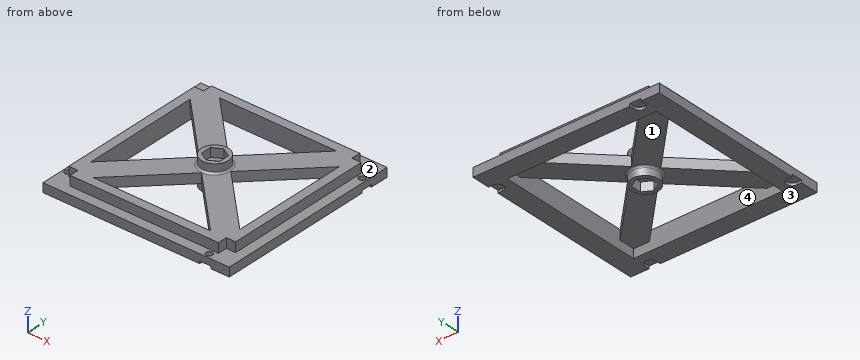
```python
from build123d import *

# Parameters (mm, degrees)
SKETCH_W           = 100
SKETCH_H           = 100
SKETCH_W_2         = 80
SKETCH_H_2         = 80
PAD_DEPTH          = 4.8
SKETCH001_R        = 2.75
PAD001_DEPTH       = 5.2
SKETCH002_R        = 7.25
PAD002_DEPTH       = 4.8
SKETCH003_R        = 7.25
PAD003_DEPTH       = 4.8
POCKET001_DEPTH    = 1.3
SKETCH006_R        = 1.75
POCKET002_DEPTH    = 3.49
POLARPATTERN_COUNT = 4
FILLET_R           = 1


with BuildPart() as part:
    # Sketch → Pad (new body)
    with BuildSketch(Plane.XY):
        Rectangle(SKETCH_W, SKETCH_H)
        Rectangle(SKETCH_W_2, SKETCH_H_2, mode=Mode.SUBTRACT)
    extrude(amount=PAD_DEPTH)

    # Sketch001 (on Face10 of Pad) → Pad001 (join)
    with BuildSketch(Plane.XY.offset(4.8)):
        Polygon((-44.8, 39.8), (-44.8, -39.8), (-39.8, -39.8), (-39.8, -44.8), (39.8, -44.8), (39.8, -39.8), (44.8, -39.8), (44.8, 39.8), (39.8, 39.8), (39.8, 44.8), (-39.8, 44.8), (-39.8, 39.8), align=None)
        Circle(SKETCH001_R, mode=Mode.SUBTRACT)
        Polygon((-31.5, 40), (0, 8.5), (31.5, 40), align=None, mode=Mode.SUBTRACT)
        Polygon((-40, 31.5), (-8.5, 0), (-40, -31.5), align=None, mode=Mode.SUBTRACT)
        Polygon((8.5, 0), (40, 31.5), (40, -31.5), align=None, mode=Mode.SUBTRACT)
        Polygon((0, -8.5), (31.5, -40), (-31.5, -40), align=None, mode=Mode.SUBTRACT)
    extrude(amount=PAD001_DEPTH)

    # Sketch002 (on Face20 of Pad001) → Pad002 (join)
    with BuildSketch(Plane.XY.offset(10)):
        Circle(SKETCH002_R)
        Polygon((0, -5.658033), (4.9, -2.829016), (4.9, 2.829016), (0, 5.658033), (-4.9, 2.829016), (-4.9, -2.829016), align=None, mode=Mode.SUBTRACT)
    extrude(amount=PAD002_DEPTH)

    # Sketch003 (on Face23 of Pad002) → Pad003 (join)
    with BuildSketch(Plane(origin=(0, 0, 4.8), x_dir=(1, 0, 0), z_dir=(0, 0, -1))):
        Circle(SKETCH003_R)
        Polygon((0, -5.658033), (4.9, -2.829016), (4.9, 2.829016), (0, 5.658033), (-4.9, 2.829016), (-4.9, -2.829016), align=None, mode=Mode.SUBTRACT)
    extrude(amount=PAD003_DEPTH)

    # Sketch005 → Pocket001 (cut)
    with BuildSketch(Plane(origin=(0, 0, 0), x_dir=(1, 0, 0), z_dir=(0, 0, -1))):
        with BuildLine():
            ThreePointArc((34.15, 47.5), (37.15, 44.5), (40.15, 47.5))
            Line((40.15, 50), (40.15, 47.5))
            Line((34.15, 50), (40.15, 50))
            Line((34.15, 47.5), (34.15, 50))
        make_face()
    pocket001 = extrude(amount=-POCKET001_DEPTH, mode=Mode.SUBTRACT)

    # Sketch006 (on Face5 of Pocket001) → Pocket002 (cut)
    with BuildSketch(Plane.XY.offset(4.8)):
        with Locations((37.15, -47.5)):
            Circle(SKETCH006_R)
    pocket002 = extrude(amount=-POCKET002_DEPTH, mode=Mode.SUBTRACT)

    # PolarPattern: Pocket002, Pocket001 ×4 about axis
    polarpattern_axis = Axis((0, 0, 4.8), (0, 0, 1))
    for i in range(1, POLARPATTERN_COUNT):
        add(pocket002.rotate(polarpattern_axis, i * 360 / POLARPATTERN_COUNT), mode=Mode.SUBTRACT)
        add(pocket001.rotate(polarpattern_axis, i * 360 / POLARPATTERN_COUNT), mode=Mode.SUBTRACT)

    # Fillet
    fillet_edges = [part.edges().sort_by_distance(p)[0] for p in [
        (-7.25, 0, 10),
        (-7.25, 0, 4.8),
    ]]
    fillet(fillet_edges, radius=FILLET_R)


solid = part.part
```
Input: part model. Units: mm. Frame: model coordinates. Face numbers are marked on the shaded views. A direction names the side the tool comes from. Give positions to 0.01 mm unless a question says otherwise; leave off trailing zeros. Order: outer loops, then holes, each group sorted by start corner. A loop starts at its lowest first (then second) coordinate and runs counter-clockwise, first axis right, second up. Notation, with made-up numbers: (17.5, 42.5) - (75.5, 42.5) arc R28 cw to (75.5, 72.5) - close; hole circle Ø1 at (62, 50.25). An arc over 180 degrees is marked (long way). One line per item, written item: value.
1. Line query: probe 1 along Y at (x, z) = (-37.15, 3.9); probe 2 along Y at (x, z) = (0, 6.2). Output: solid intervals per line, ascending.
Determined:
probe 1: -50 to -40, 40 to 45.75, 49.25 to 50
probe 2: -44.8 to -40, -8.5 to -2.75, 2.75 to 8.5, 40 to 44.8
2. Draft query along X for the marked faces 3 and 4. Return one class per face: released by +X, released by -X, zero draft, split by the parting line, or undercut.
Determined:
face 3: zero draft
face 4: undercut
3. Cut plane B-B, the plane z = 7.75. Output: boundary loops of the cut face in (x, y).
Determined:
outline: (-44.8, -39.8) - (-39.8, -39.8) - (-39.8, -44.8) - (39.8, -44.8) - (39.8, -39.8) - (44.8, -39.8) - (44.8, 39.8) - (39.8, 39.8) - (39.8, 44.8) - (-39.8, 44.8) - (-39.8, 39.8) - (-44.8, 39.8) - close; hole (-40, -31.5) - (-8.5, 0) - (-40, 31.5) - close; hole (-31.5, -40) - (31.5, -40) - (0, -8.5) - close; hole (-31.5, 40) - (0, 8.5) - (31.5, 40) - close; hole circle Ø5.5 at (0, 0); hole (8.5, 0) - (40, -31.5) - (40, 31.5) - close
4. Cut plane D-D, the plane x = 17. Output: boundary loops of the cut face in (y, z).
Determined:
outline: (-50, 0) - (-40, 0) - (-40, 10) - (-44.8, 10) - (-44.8, 4.8) - (-50, 4.8) - close; (-25.5, 4.8) - (-8.5, 4.8) - (-8.5, 10) - (-25.5, 10) - close; (8.5, 4.8) - (25.5, 4.8) - (25.5, 10) - (8.5, 10) - close; (40, 0) - (50, 0) - (50, 4.8) - (44.8, 4.8) - (44.8, 10) - (40, 10) - close
5. Cut plane A-A, the plane x = 37.15. Output: boundary loops of the cut face in (y, z), and give its area (3 significant figures).
Determined:
outline: (-50, 1.3) - (-44.5, 1.3) - (-44.5, 0) - (-40, 0) - (-40, 4.8) - (-28.65, 4.8) - (-28.65, 10) - (-44.8, 10) - (-44.8, 4.8) - (-45.75, 4.8) - (-45.75, 1.31) - (-49.25, 1.31) - (-49.25, 4.8) - (-50, 4.8) - close; (28.65, 4.8) - (40, 4.8) - (40, 0) - (50, 0) - (50, 4.8) - (44.8, 4.8) - (44.8, 10) - (28.65, 10) - close
area: 245 mm2
6. Cut plane C-C, the plane y = 37.15. Output: boundary loops of the cut face in (x, z), and give its area (3 significant figures).
Determined:
outline: (-50, 0) - (-40, 0) - (-40, 4.8) - (-28.65, 4.8) - (-28.65, 10) - (-44.8, 10) - (-44.8, 4.8) - (-50, 4.8) - close; (28.65, 4.8) - (40, 4.8) - (40, 0) - (44.5, 0) - (44.5, 1.3) - (50, 1.3) - (50, 4.8) - (49.25, 4.8) - (49.25, 1.31) - (45.75, 1.31) - (45.75, 4.8) - (44.8, 4.8) - (44.8, 10) - (28.65, 10) - close
area: 245 mm2
7. Reachability of the marked faces 1 and 2 from +Z, -Z, +X, -X, +Y, -Y: full face, straight path, thin tool, end or side. Return the list, or none.
Determined:
face 1: -Z
face 2: +Z
8. Pin query (flat end, axial travel): pin 1 Ø3 at (x, y) = (-47, -37) entering from +Z; pin 2 Ø5.5 at (x, y) = (-37.15, 47.5) entering from +Z; pin 3 Ø2.5 at (x, z) = (-42, 7) entering from -Y. Return the tip coordinate at first contact, or that it passes through.
Determined:
pin 1: z = 4.8
pin 2: z = 10
pin 3: y = -39.8
